from build123d import *

# Parameters (mm, degrees)
SKETCH1_W            = 64.75
SKETCH1_H            = 20
BODY_DEPTH           = 140
SHELL1_T             = 3
SWITCH_CUTOUT_REACH  = 148.722
SKETCH2_W            = 26.75
SKETCH2_H            = 12
SKETCH4_W            = 15
SKETCH4_H            = 27
SKETCH4_R            = 4.0125
AXLE_HOLDER_DEPTH    = 15
SKETCH5_R            = 4.0125
SKETCH5_R_2          = 2.5
BUSHING_HOLDER_DEPTH = 9
FILLET3_R            = 4
FILLET4_R            = 6
SKETCH6_W            = 125
SKETCH6_H            = 10
SLIDE_MOUNT_DEPTH    = 3.5
CIRPATTERN1_COUNT    = 2
FILLET6_R            = 3
FILLET7_R            = 3
FILLET8_R            = 6
CUT_EXTRUDE1_REACH   = 147.177
SKETCH7_R            = 5
SKETCH8_R            = 9.916079783
CUT_EXTRUDE2_DEPTH   = 9
CUT_EXTRUDE3_DEPTH   = 3.5


with BuildPart() as part:
    # Sketch1 → Body (new body)
    with BuildSketch(Plane.XY):
        Rectangle(SKETCH1_W, SKETCH1_H)
    extrude(amount=BODY_DEPTH)

    # Shell1
    shell1_openings = [part.faces().sort_by_distance(p)[0] for p in [
        (0, 0, 0),
        (0, 0, 140),
    ]]
    offset(amount=SHELL1_T, openings=shell1_openings, kind=Kind.INTERSECTION)

    # Sketch2 → Switch_cutout (cut, up to next)
    with BuildSketch(Plane(origin=(0, 13, 0), x_dir=(1, 0, 0), z_dir=(0, 1, 0)), mode=Mode.PRIVATE) as switch_cutout_sk1:
        with Locations((18, -6)):
            Rectangle(SKETCH2_W, SKETCH2_H)
    switch_cutout_tool1 = extrude(switch_cutout_sk1.sketch, amount=-SWITCH_CUTOUT_REACH, mode=Mode.PRIVATE) & part.part
    # Sketch2 → Switch_cutout (cut, up to next)
    with BuildSketch(Plane(origin=(0, 13, 0), x_dir=(1, 0, 0), z_dir=(0, 1, 0)), mode=Mode.PRIVATE) as switch_cutout_sk2:
        with Locations((-18, -134)):
            Rectangle(SKETCH2_W, SKETCH2_H)
    switch_cutout_tool2 = extrude(switch_cutout_sk2.sketch, amount=-SWITCH_CUTOUT_REACH, mode=Mode.PRIVATE) & part.part
    add(switch_cutout_tool1.solids().sort_by_distance((18, 13, 6))[0], mode=Mode.SUBTRACT)
    add(switch_cutout_tool2.solids().sort_by_distance((-18, 13, 134))[0], mode=Mode.SUBTRACT)

    # Sketch4 → Axle_holder (add, symmetric)
    # profile 1 of 2: a face of its own
    with BuildSketch(Plane.ZY):
        with Locations((12.5, -26.5)):
            Rectangle(SKETCH4_W, SKETCH4_H)
        with Locations(Location((12.5, -32.5, 0), (0, 0, 270))):
            Circle(SKETCH4_R, mode=Mode.SUBTRACT)
    # profile 2 of 2: a face of its own
    with BuildSketch(Plane.ZY):
        with Locations((127.5, -26.5)):
            Rectangle(SKETCH4_W, SKETCH4_H)
        with Locations(Location((127.5, -32.5, 0), (0, 0, 90))):
            Circle(SKETCH4_R, mode=Mode.SUBTRACT)
    extrude(amount=AXLE_HOLDER_DEPTH, both=True)

    # Sketch5 → Bushing_holder (add, symmetric)
    # profile 1 of 2: a face of its own
    with BuildSketch(Plane.ZY):
        with Locations(Location((12.5, -32.5, 0), (0, 0, 270))):
            Circle(SKETCH5_R)
        with Locations(Location((12.5, -32.5, 0), (0, 0, 270))):
            Circle(SKETCH5_R_2, mode=Mode.SUBTRACT)
    # profile 2 of 2: a face of its own
    with BuildSketch(Plane.ZY):
        with Locations(Location((127.5, -32.5, 0), (0, 0, 90))):
            Circle(SKETCH5_R)
        with Locations(Location((127.5, -32.5, 0), (0, 0, 270))):
            Circle(SKETCH5_R_2, mode=Mode.SUBTRACT)
    extrude(amount=BUSHING_HOLDER_DEPTH, both=True)

    # Fillet3
    fillet3_edges = [part.edges().sort_by_distance(p)[0] for p in [
        (0, -40, 5),
        (0, -40, 20),
        (0, -40, 135),
        (0, -40, 120),
    ]]
    fillet(fillet3_edges, radius=FILLET3_R)

    # Fillet4
    # the kernel refuses this fillet: 6 mm, written as the material it adds along each edge
    with BuildSketch(Plane(origin=(15, -13, 5), x_dir=(0, 0, -1), z_dir=(-1, 0, 0))) as fillet4_piece_1:
        with BuildLine():
            CenterArc((6, 5.916079783), FILLET4_R, 180, 80.405931773)
            Line((0, 5.916079783), (-0.12, 5.916079783))
            Line((-0.12, 5.916079783), (-0.12, 0))
            Line((-0.12, 0), (0, -0.12))
            ThreePointArc((0, -0.12), (2.5, -0.12), (4.98, -0.118321596))
            Line((4.98, -0.118321596), (5, 0))
        make_face()
    extrude(amount=30)
    with BuildSketch(Plane(origin=(-15, -13, 20), x_dir=(0, 0, 1), z_dir=(1, 0, 0)), Plane(origin=(-15, -13, 120), x_dir=(0, -1, 0), z_dir=(1, 0, 0))) as fillet4_piece_2:
        with BuildLine():
            CenterArc((FILLET4_R, FILLET4_R), FILLET4_R, 180, 90)
            Line((0, FILLET4_R), (-FILLET4_R * 0.02, FILLET4_R))
            Line((-FILLET4_R * 0.02, FILLET4_R), (-FILLET4_R * 0.02, -FILLET4_R * 0.02))
            Line((-FILLET4_R * 0.02, -FILLET4_R * 0.02), (FILLET4_R, -FILLET4_R * 0.02))
            Line((FILLET4_R, -FILLET4_R * 0.02), (FILLET4_R, 0))
        make_face()
    extrude(amount=30)
    with BuildSketch(Plane(origin=(15, -13, 135), x_dir=(0, 0, 1), z_dir=(-1, 0, 0))) as fillet4_piece_3:
        with BuildLine():
            CenterArc((6, -5.916079783), FILLET4_R, 99.594068227, 80.405931773)
            Line((0, -5.916079783), (-0.12, -5.916079783))
            Line((-0.12, -5.916079783), (-0.12, 0))
            Line((-0.12, 0), (0, 0.12))
            ThreePointArc((0, 0.12), (2.5, 0.12), (4.98, 0.118321596))
            Line((4.98, 0.118321596), (5, 0))
        make_face()
    extrude(amount=30)

    # Sketch6 → Slide_mount (add)
    with BuildSketch(Plane(origin=(35.375, 0, 0), x_dir=(0, 0, -1), z_dir=(1, 0, 0))):
        with Locations((-77.5, 18)):
            Rectangle(SKETCH6_W, SKETCH6_H)
        with BuildLine():
            Line((-135, 18.7), (-20, 18.7))
            ThreePointArc((-20, 18.7), (-18.3, 17), (-20, 15.3))
            Line((-20, 15.3), (-135, 15.3))
            ThreePointArc((-135, 15.3), (-136.7, 17), (-135, 18.7))
        make_face(mode=Mode.SUBTRACT)
    slide_mount = extrude(amount=-SLIDE_MOUNT_DEPTH)

    # CirPattern1: Slide_mount ×2 about axis
    cirpattern1_axis = Axis((0, 0, 70), (0, 1, 0))
    for i in range(1, CIRPATTERN1_COUNT):
        add(slide_mount.rotate(cirpattern1_axis, i * 360 / CIRPATTERN1_COUNT))

    # Fillet6
    fillet6_edges = [part.edges().sort_by_distance(p)[0] for p in [
        (33.625, 23, 140),
        (33.625, 23, 15),
        (-33.625, 23, 0),
        (-33.625, 23, 125),
    ]]
    fillet(fillet6_edges, radius=FILLET6_R)

    # Fillet7
    fillet7_edges = [part.edges().sort_by_distance(p)[0] for p in [
        (4.625, 11.5, 12),
        (31.375, 11.5, 12),
        (-31.375, 11.5, 128),
        (-4.625, 11.5, 128),
    ]]
    fillet(fillet7_edges, radius=FILLET7_R)

    # Fillet8
    fillet8_edges = [part.edges().sort_by_distance(p)[0] for p in [
        (33.625, 13, 15),
        (-33.625, 13, 125),
    ]]
    fillet(fillet8_edges, radius=FILLET8_R)

    # Sketch7 → Cut-Extrude1 (cut, up to next)
    with BuildSketch(Plane.XY.offset(135), mode=Mode.PRIVATE) as cut_extrude1_sk1:
        with Locations(Location((0, -22.916079783, 0), (0, 0, 51.555975818))):
            Circle(SKETCH7_R)
    cut_extrude1_tool1 = extrude(cut_extrude1_sk1.sketch, amount=-CUT_EXTRUDE1_REACH, mode=Mode.PRIVATE) & part.part
    add(cut_extrude1_tool1.solids().sort_by_distance((0, -22.91608, 135))[0], mode=Mode.SUBTRACT)

    # Sketch8 → Cut-Extrude2 (cut)
    with BuildSketch(Plane.XY.offset(135)):
        with Locations((0, -22.916079783)):
            Circle(SKETCH8_R)
    extrude(amount=CUT_EXTRUDE2_DEPTH, mode=Mode.SUBTRACT)

    # Sketch9 → Cut-Extrude3 (cut, symmetric)
    with BuildSketch(Plane(origin=(0, 0, 120), x_dir=(-1, 0, 0), z_dir=(0, 0, -1))):
        Polygon((-6.697263123, -22.916079783), (-3.348631561, -28.716079783), (3.348631561, -28.716079783), (6.697263123, -22.916079783), (3.348631561, -17.116079783), (-3.348631561, -17.116079783), align=None)
    extrude(amount=CUT_EXTRUDE3_DEPTH, both=True, mode=Mode.SUBTRACT)


solid = part.part
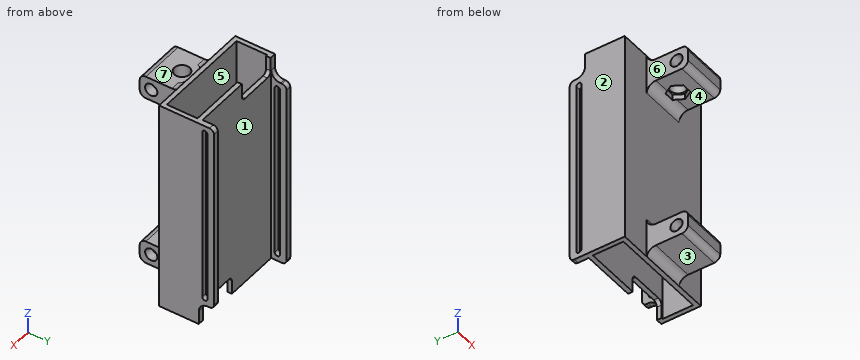
Design review of the part built by this model. Coordinates are the model's own, in mm. Face numbers are marked on the shaded views. A direction names the side the tool comes from. Coordinates: 2 decimals unless noted, no trailing zeros. Write each loop counter-clockwise with the first axis right and the second up, starting at its lowest first coordinate (ties: lowest second). Pieces come first, ordered by that corner, then holes. Notation, with made-up numbers: (-4.5, -27) - (-0.5, -27) arc R12 ccw to (-0.5, -6) - close; hole circle Ø7 at (-24, 67). An arc over 180 degrees is marked (long way). One line per item, written item: value.
1) For the marked faces 4, 5, 6 and 7, list the 3-axis set-ups (+Z, -Z, +X, -X, +Y, -Y) from which the entire face can be reached by the end or side of a thin tool; tool diameter is ignored.
Answer sheet:
face 4: +X, -X, -Y
face 5: +Z, -Z
face 6: +Z, -Z, -X, -Y
face 7: +Z, -Y
2) To check wall thickness, follow probe 1 along Z at (x, y) = (-10.4, -32.5); probe 2 along Y at (x, z) = (-4.5, 68); probe 3 along Z at (x, y) = (5, -32). State the ranges of each line that lie inside material, in increasing order.
Answer sheet:
probe 1: z = 5 to 8.49, 16.51 to 20, 120 to 123.49, 131.51 to 135
probe 2: y = -13 to -10, 10 to 13
probe 3: z = 5 to 10.05, 14.95 to 20, 120 to 125.05, 129.95 to 135
3) Add section C-C (x = -24.5). State the section outline as (y, z) points.
Answer sheet:
outline: (-13, 0) - (-10, 0) - (-10, 140) - (-13, 140) - close; (10, 0) - (13, 0) - (13, 128) - (10, 128) - close
4) Insertion check: pin 1 (10 mm diameter, centred on x = -20.5, z = 110, fed in from +Y); pin 2 (21 mm diameter, centred on x = 10, z = 47, fed in from -Y); pin 3 (9.5 mm diameter, centred on x = -0.5, y = -26, fed in from -Z). Each pin has a flat end and moves straight along its axis. Give the tip position at first contact, or say it passes through.
Answer sheet:
pin 1: stops at y = 13
pin 2: stops at y = -13
pin 3: stops at z = 5
5) Mouldability with a two-part tool opening along X and no side actions: class the marked faces 1, 2 and 3 as +X half, -X half, draft (parallel to the pull), parting line (faces both ways), or undercut.
Answer sheet:
face 1: undercut
face 2: -X half
face 3: draft
6) Add section D-D (y = -2). State the section outline as (x, z) points (3 decimals).
Answer sheet:
outline: (-35.375, 0) - (-32.375, 0) - (-32.375, 140) - (-35.375, 140) - close; (32.375, 0) - (35.375, 0) - (35.375, 140) - (32.375, 140) - close
7) Add section B-B (y = -32.5). Give the number of separate pieces and of enclosed holes in the cut face, plus the area to 3 significant figures.
Answer sheet:
separate pieces: 4
enclosed holes: 0
area: 527 mm2
8) Add section A-A (z = 48.5). State the section outline as (x, y) points (3 decimals), plus the area to 3 significant figures.
Answer sheet:
outline: (-35.375, -13) - (35.375, -13) - (35.375, 15.3) - (31.875, 15.3) - (31.875, 13) - (-31.875, 13) - (-31.875, 15.3) - (-35.375, 15.3) - close; (-35.375, 18.7) - (-31.875, 18.7) - (-31.875, 23) - (-35.375, 23) - close; (31.875, 18.7) - (35.375, 18.7) - (35.375, 23) - (31.875, 23) - close; hole (-32.375, -10) - (32.375, -10) - (32.375, 10) - (-32.375, 10) - close
area: 591 mm2
